For this review, take the finished solid that the model builds, in its own axes (mm). A direction names the side the tool comes from. Coordinates: 2 decimals unless noted, no trailing zeros. Order: outer loops, then holes, each group sorted by start corner. A loop starts at its lowest first (then second) coordinate and runs counter-clockwise, first axis right, second up.
Autodesk Inventor part; units mm, degrees
ref_plane "YZ Plane" through (0, 0, 0) normal (1, 0, 0) x (0, 1, 0)
ref_plane "XZ Plane" through (0, 0, 0) normal (0, 1, 0) x (-1, 0, 0)
ref_plane "XY Plane" through (0, 0, 0) normal (0, 0, 1) x (1, 0, 0)
sketch "Boceto1" plane through (0, 0, 0) normal (0, 1, 0) x (-1, 0, 0)
  circle A0 centre (0, 0) radius 90
  dimension "d0" = 180
extrude "Extrusión1" add sketch "Boceto1" along normal blind 15
extrude "Extrusión2" add sketch "Boceto1" against normal blind 25 draft -45
shell "Vaciado1" thickness 1 removed faces 1 at (19.6237, 15, 24.7178)
sketch "Boceto2" plane through (0, -25, 0) normal (0, -1, 0) x (1, 0, 0)
  circle A0 centre (0, 0) radius 12.5
  dimension "d6" = 25
extrude "Extrusión3" cut sketch "Boceto2" against normal blind 25
sketch "Boceto3" plane through (0, -25, 0) normal (0, -1, 0) x (1, 0, 0)
  circle A0 centre (0, 0) radius 12.5
  circle A1 centre (0, 0) radius 45
  circle A2 centre (0, 0) radius 44
  line L0 (44, 0) -> (41.5, 0)
  circle A3 centre (41.5, 0) radius 2.5
  line L1 (-44, 0) -> (-41.5, 0)
  circle A4 centre (-41.5, 0) radius 2.5
  circle A5 centre (0, 41.5) radius 2.5
  circle A6 centre (-41.5, 0) radius 2.5
  circle A7 centre (0, -41.5) radius 2.5
  line L2 (44, 0) -> (39, 0)
  circle A8 centre (39, 0) radius 5
  circle A9 centre (-39, 0) radius 5
  point P0 (0, 44)
  point P1 (-44, 0)
  point P2 (0, -44)
  dimension "d9" = 90
  dimension "d10" = 88
  dimension "d11" = 2.5
  dimension "d12" = 2.5
  dimension "d13" = 5
  dimension "d16" = 360
extrude "Extrusión4" add sketch "Boceto3" along normal blind 450 contours A4 | A9 | A3 L2 L0 | L0 L2 A3 | A8
shell "Vaciado2" thickness 1 removed faces 2 at (-39.591, -475, 0.7606) at (39.8768, -475, -0.3989)
properties part number "base"
1. Machinability: for faces 5 (the face through (11.923, -24.507, 3.755)), 6 (the face through (34, -247, 0)), 7 (the face through (-13, -24, 1)), which of the approach directions +Z, -Z, +X, -X, +Y, -Y give a long, thin tool a straight path to every point of the face, cutting with its end or side? Answer none if there is none.
Answer below:
face 5: +Y, -Y
face 6: -Y
face 7: +Y
2. Take a section at B-B, the plane y = -424. Give the boundary of the cut face in (x, z).
Answer below:
outline: circle Ø10 at (-39, 0); circle Ø10 at (39, 0); hole circle Ø8 at (-39, 0); hole circle Ø8 at (39, 0)
3. To check wall thickness, follow L1, parallel to Z at x = 39, y = -381; L2, parallel to Y at x = -49.5, z = 26; L3, parallel to Y at x = 48, z = 66. State the ranges of each line that lie inside material, in increasing order.
Answer below:
L1: z = -5 to -4, 4 to 5
L2: y = -25 to -24
L3: y = -8.39 to -6.98
4. Clearance check with flat-ended pins moving along their axes: pin 1 Ø5 at (x, z) = (39, 0) entering from -Y; pin 2 Ø8 at (y, z) = (-212.5, 1.5) entering from +X; pin 3 Ø5 at (x, z) = (-39, 0) entering from +Y. State where each tip first meets the part, or that it passes through.
Answer below:
pin 1: stops at y = -25
pin 2: stops at x = 44
pin 3: stops at y = -24
5. Take a section at A-A, the plane x = 0. Give the boundary of the cut face in (y, z).
Answer below:
outline: (-25, -65) - (0, -90) - (15, -90) - (15, -89) - (0.41, -89) - (-24, -64.59) - (-24, -12.5) - (-25, -12.5) - close; (-25, 12.5) - (-24, 12.5) - (-24, 64.59) - (0.41, 89) - (15, 89) - (15, 90) - (0, 90) - (-25, 65) - close
6. The part is to be moulded in two halves that separate along Z. For faces 1 (the face through (-44, -247, 0)), 2 (the face through (65.597, 7.605, -60.15)), 3 (the face through (87, 15, 20)), 4 (the face through (14.332, -22.473, -64.541)), say which applies: +Z half, -Z half, draft (parallel to the pull), parting line (faces both ways), or undercut.
Answer below:
face 1: parting line
face 2: undercut
face 3: draft
face 4: undercut
